from build123d import *

# Parameters (mm, degrees)
SKETCH_R  = 3.5
PAD_DEPTH = 2


with BuildPart() as part:
    # Sketch → Pad (new body)
    with BuildSketch(Plane.XY):
        with BuildLine():
            ThreePointArc((-22.5, 8), (-30.5, 0), (-22.5, -8))
            Line((-22.5, -8), (22.5, -8))
            ThreePointArc((22.5, -8), (30.5, 0), (22.5, 8))
            Line((-22.5, 8), (22.5, 8))
        make_face()
        with Locations((-22.5, 0)):
            Circle(SKETCH_R, mode=Mode.SUBTRACT)
        with Locations((22.5, 0)):
            Circle(SKETCH_R, mode=Mode.SUBTRACT)
        with Locations((-7.5, 0)):
            Circle(SKETCH_R, mode=Mode.SUBTRACT)
        with Locations((7.5, 0)):
            Circle(SKETCH_R, mode=Mode.SUBTRACT)
    extrude(amount=PAD_DEPTH)


solid = part.part
Work out the finished part from the listing and answer in its coordinate system (mm). Round coordinates to 2 decimals unless told otherwise and drop trailing zeros. Loops run counter-clockwise (first coordinate to the right, second up) from the corner with the lowest first, then second, coordinate; pieces in that order, holes last. Notation, with made-up numbers: (25.25, 62.25) - (55.25, 62.25) arc R21 ccw to (55.25, 99.25) - close; hole circle Ø4 at (38.25, 30). An arc over 180 degrees is marked (long way). One line per item, written item: value.
Q1. Find section C-C on x = 7.5. Give the vertices of the cut face in (y, z).
Check values:
outline: (-8, 0) - (-3.5, 0) - (-3.5, 2) - (-8, 2) - close; (3.5, 0) - (8, 0) - (8, 2) - (3.5, 2) - close
Q2. Find section D-D on y = 2.75. Give the vertices of the cut face in (x, z).
Check values:
outline: (-30.01, 0) - (-24.67, 0) - (-24.67, 2) - (-30.01, 2) - close; (-20.33, 0) - (-9.67, 0) - (-9.67, 2) - (-20.33, 2) - close; (-5.33, 0) - (5.33, 0) - (5.33, 2) - (-5.33, 2) - close; (9.67, 0) - (20.33, 0) - (20.33, 2) - (9.67, 2) - close; (24.67, 0) - (30.01, 0) - (30.01, 2) - (24.67, 2) - close
Q3. Find section B-B on z = 0.5. Give the vertices of the cut face in (x, y).
Check values:
outline: (-22.5, -8) - (22.5, -8) arc R8 ccw to (22.5, 8) - (-22.5, 8) arc R8 ccw to start; hole circle Ø7 at (-22.5, 0); hole circle Ø7 at (-7.5, 0); hole circle Ø7 at (7.5, 0); hole circle Ø7 at (22.5, 0)
Q4. The mould has two halves that part along Y. Classify faces 1 (the flat face through (0, 0, 0)), 2 (the cylindrical face through (-19.16, 1.05, 0.99)), 3 (the cylindrical face through (-30.498, 0.176, 0.986)), 4 (the cylindrical face through (-11, 0, 1)): +Y half, -Y half, draft (parallel to the pull), parting line (faces both ways), or undercut.
Check values:
face 1: draft
face 2: undercut
face 3: parting line
face 4: undercut
Q5. Find section A-A on y = 0. Give the vertices of the cut face in (x, z), and give its area (3 significant figures).
Check values:
outline: (-30.5, 0) - (-26, 0) - (-26, 2) - (-30.5, 2) - close; (-19, 0) - (-11, 0) - (-11, 2) - (-19, 2) - close; (-4, 0) - (4, 0) - (4, 2) - (-4, 2) - close; (11, 0) - (19, 0) - (19, 2) - (11, 2) - close; (26, 0) - (30.5, 0) - (30.5, 2) - (26, 2) - close
area: 66.0 mm2
Q6. Each of these flat-tipped pins is pushed along its axis until it touches: pin 1 Ø9 at (x, y) = (-22.5, 0) entering from -Z; pin 2 Ø1 at (y, z) = (-5, 0.5) entering from -X. Where does it stop, or does it pass through?
Check values:
pin 1: z = 0
pin 2: x = -29.11
Q7. Straight lines are drawn through the part: probe 1 along Y at (x, z) = (-22.5, 1.45); probe 2 along X at (y, z) = (1.5, 0.2); probe 3 along X at (y, z) = (2.5, 1.4). For each, find the intervals that lie inside material, in ascending order.
Check values:
probe 1: -8 to -3.5, 3.5 to 8
probe 2: -30.36 to -25.66, -19.34 to -10.66, -4.34 to 4.34, 10.66 to 19.34, 25.66 to 30.36
probe 3: -30.1 to -24.95, -20.05 to -9.95, -5.05 to 5.05, 9.95 to 20.05, 24.95 to 30.1
